```python
from build123d import *

# Parameters (mm, degrees)
F2_R = 0.682367
F3_R = 8.749241


with BuildPart() as f1:
    # F0 (on Front) → F1 (revolve)
    with BuildSketch(Plane.XZ):
        Polygon((0, 11.625385), (0, 0), (3.367648, 7.997596), (11.65795, 11.625385), align=None)
    revolve(axis=Axis((0, 0, 5.812692), (0, 0, -1)))

    # F2
    f2_edges = [f1.edges().sort_by_distance(p)[0] for p in [
        (-11.65795, 0, 11.625385),
    ]]
    fillet(f2_edges, radius=F2_R)

    # F3
    f3_edges = [f1.edges().sort_by_distance(p)[0] for p in [
        (-3.367648, 0, 7.997596),
    ]]
    fillet(f3_edges, radius=F3_R)


solid = f1.part
```
Build history of the part. All positions in model axes, mm. Coordinates: 2 decimals unless noted, no trailing zeros. Order: outer loops, then holes, each group sorted by start corner. A loop starts at its lowest first (then second) coordinate and runs counter-clockwise, first axis right, second up.
Item 1: Drill centre lines: L1, parallel to Z at x = 3.5, y = -7; L2, parallel to Z at x = 0.25, y = 6; L3, parallel to X at y = -0.5, z = 7.75. Where is each one in solid material? Low to high.
Filled in:
L1: z = 9.95 to 11.63
L2: z = 9.13 to 11.63
L3: x = -4.04 to 4.04
Item 2: Saw through at B-B on z = 4.5. List the corners of the cut face in (x, y).
Filled in:
outline: circle Ø3.79 at (0, 0)
Item 3: Saw through at A-A on z = 1. List the corners of the cut face in (x, y), then the cut area to 3 significant figures.
Filled in:
outline: circle Ø0.84 at (0, 0)
area: 0.557 mm2
Item 4: Drop a flat-ended pin along its axis: pin 1 Ø1.5 at (y, z) = (0.5, 10) entering from +X. Give the stop position or say it passes through.
Filled in:
pin 1: stops at x = 9.04
